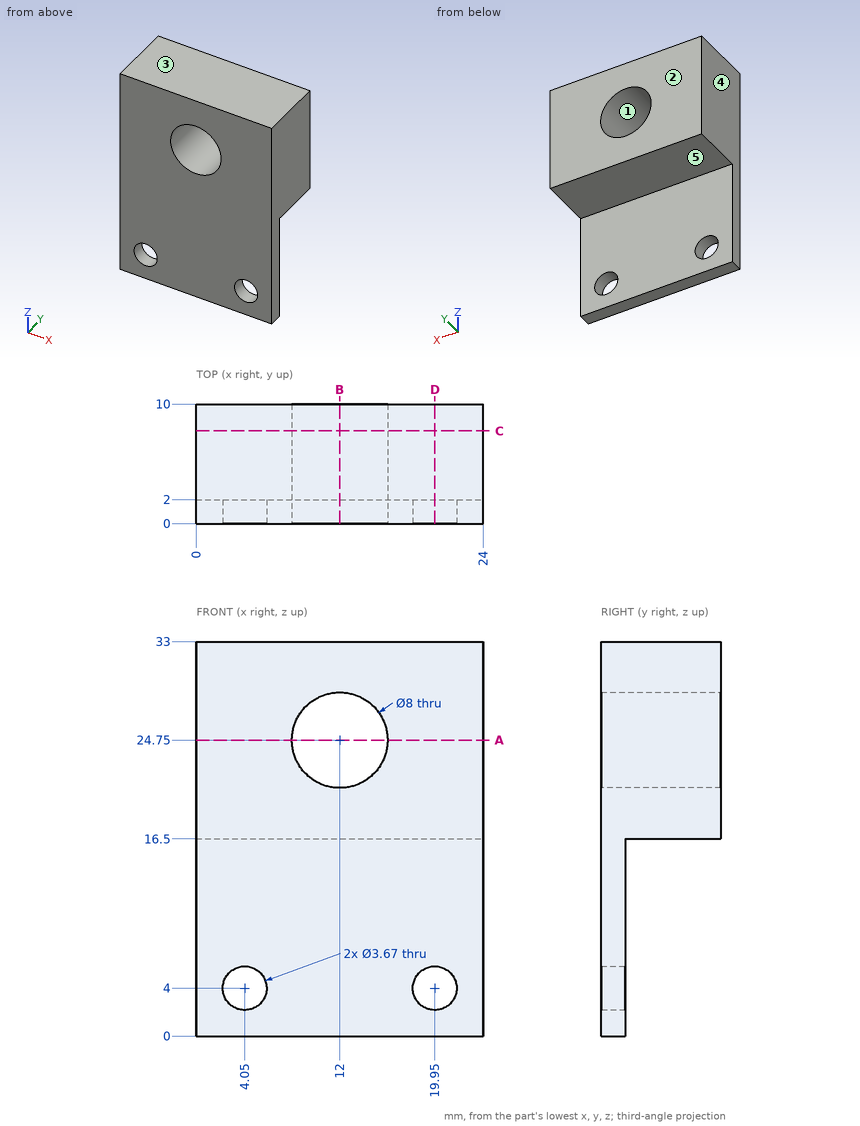
Drawing for the job (mm, zero at the part's lowest x, y, z). A direction names the side the tool comes from. Give positions to 0.01 mm unless a question says otherwise; leave off trailing zeros. Order: outer loops, then holes, each group sorted by start corner. A loop starts at its lowest first (then second) coordinate and runs counter-clockwise, first axis right, second up. Notation, with made-up numbers: M 80.5,45.5 L 135.5,45.5 A26 ccw 135.5,68.5 Z; hole C 31.5,87 d4. An arc over 180 degrees is marked long. Put each result on its own line as item: value. Start each with the question number.
(1) Saw through at C-C, the plane y = 7.75. Write the cut outline in (x, z).
(2) Saw through at B-B, the plane x = 12. Write the cut outline in (y, z).
(3) Saw through at D-D, the plane x = 19.95. Write the cut outline in (y, z) (3 decimals).
(4) Which spindle directions (+Z, -Z, +X, -X, +Y, -Y) get a long thin tool onto all of the face, cutting with end or side? Do the marked faces 4 and 5. Say none if no direction does.
(5) Saw through at A-A, the plane z = 24.75. Write the cut outline in (x, y), then the cut area to 3 significant figures.
(6) Mould opens along Z. For the marked faces 1, 2 and 3 say: +Z half, -Z half, draft (parallel to the pull), parting line (faces both ways), or undercut.
(7) Flat gauge pins, fed straight in: pin 1 Ø5 at (x, z) = (14.5, 6.5) entering from +Y; pin 2 Ø3 at (x, y) = (13.5, 4) entering from -Z; pin 3 Ø7 at (x, z) = (12, 24.75) entering from +Y. Where does each tip first touch, or does it go through?
(8) Drill centre lines: line 1 along X through (y, z) = (0.8, 4) (3 decimals); line 2 along Y through (x, z) = (18.25, 5); line 3 along X through (y, z) = (6.25, 25). Where is each one in solid material? Low to high.
Check result:
1. outline: M 0,16.5 L 24,16.5 L 24,33 L 0,33 Z; hole C 12,24.75 d8
2. outline: M 0,0 L 2,0 L 2,16.5 L 10,16.5 L 10,20.75 L 0,20.75 Z; M 0,28.75 L 10,28.75 L 10,33 L 0,33 Z
3. outline: M 0,0 L 2,0 L 2,2.165 L 0,2.165 Z; M 0,5.835 L 2,5.835 L 2,16.5 L 10,16.5 L 10,33 L 0,33 Z
4. face 4: +Z, -Z, -X, +Y, -Y
4. face 5: -Z, +X, -X, +Y
5. outline: M 0,0 L 8,0 L 8,10 L 0,10 Z; M 16,0 L 24,0 L 24,10 L 16,10 Z
5. area: 160 mm2
6. face 1: undercut
6. face 2: draft
6. face 3: +Z half
7. pin 1: stops at y = 2
7. pin 2: stops at z = 16.5
7. pin 3: passes through
8. line 1: x = 0 to 2.215, 5.885 to 18.115, 21.785 to 24
8. line 2: y = 0 to 2
8. line 3: x = 0 to 8.01, 15.99 to 24
